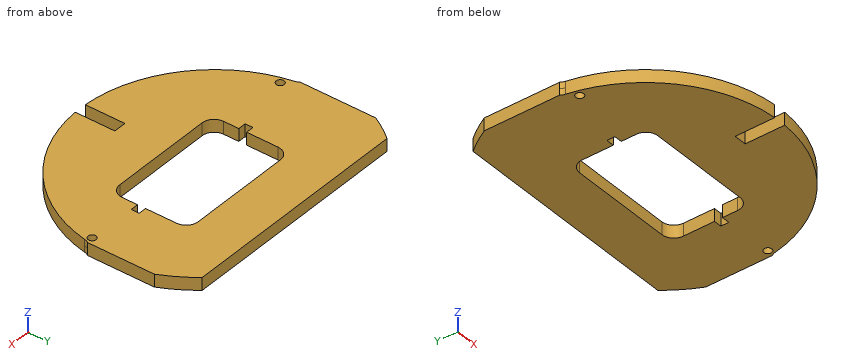
from build123d import *

# Parameters (mm, degrees)
BOSS_EXTRUDE1_DEPTH = 1.5875
SKETCH2_R           = 1
CUT_EXTRUDE1_DEPTH  = 3.175
SKETCH3_W           = 3.175
SKETCH3_H           = 10.970571453
CUT_EXTRUDE2_DEPTH  = 48.905462264
SKETCH4_W           = 2
SKETCH4_H           = 2
CUT_EXTRUDE3_DEPTH  = 48.879683973


with BuildPart() as part:
    # Sketch1 → Boss-Extrude1 (new, symmetric)
    with BuildSketch(Plane.XY):
        with BuildLine():
            Line((-29.861047016, 19.799597713), (28.798323584, 19.799597713))
            ThreePointArc((28.798323584, 19.799597713), (31.555543196, 15.909935232), (33.800017398, 11.703503281))
            Line((33.800017398, 11.703503281), (33.800017398, -5.129281896))
            add(Edge.make_bspline(
                [(33.333736062, -6.198908202), (33.370273649, -6.00495249), (33.420827163, -5.815771167), (33.570327065, -5.45389308), (33.6709127, -5.28028559), (33.800017398, -5.129281896)],
                knots=[0, 0, 0, 0, 0.5, 0.5, 1, 1, 1, 1], degree=3))
            ThreePointArc((33.333736062, -6.198908202), (-0.00068987, -33.79957838), (-33.333992426, -6.197552493))
            add(Edge.make_bspline(
                [(-33.800017403, -5.129281896), (-33.542046516, -5.431010319), (-33.407261527, -5.809359873), (-33.333992426, -6.197552493)],
                knots=[0, 0, 0, 0, 1, 1, 1, 1], degree=3))
            Line((-33.800017403, -5.129281896), (-33.800017403, 13.855371896))
            ThreePointArc((-33.800017403, 13.855371896), (-31.971328776, 16.92078434), (-29.861047016, 19.799597713))
        make_face()
    extrude(amount=BOSS_EXTRUDE1_DEPTH, both=True)

    # Sketch2 → Cut-Extrude1 (cut)
    with BuildSketch(Plane.XY.offset(1.5875)):
        with Locations((-31.216064399, -8.164436653)):
            Circle(SKETCH2_R)
        with Locations((32.009302375, -5.358989516)):
            Circle(SKETCH2_R)
    extrude(amount=-CUT_EXTRUDE1_DEPTH, mode=Mode.SUBTRACT)

    # Sketch3 → Cut-Extrude2 (cut, through all)
    with BuildSketch(Plane.XY.offset(1.5875)):
        with Locations((-0.013127042, -29.284890239)):
            Rectangle(SKETCH3_W, SKETCH3_H)
    extrude(amount=-CUT_EXTRUDE2_DEPTH, mode=Mode.SUBTRACT)

    # Sketch4 → Cut-Extrude3 (cut, through all)
    with BuildSketch(Plane.XY.offset(1.5875)):
        with BuildLine():
            Line((-14.257724699, 4.717183699), (-14.257724699, -8.984256283))
            ThreePointArc((-14.257724699, -8.984256283), (-13.379045042, -11.105576627), (-11.257724699, -11.984256283))
            Line((-11.257724699, -11.984256283), (14.878600613, -11.984256283))
            ThreePointArc((14.878600613, -11.984256283), (16.999920956, -11.105576627), (17.878600613, -8.984256283))
            Line((17.878600613, -8.984256283), (17.878600613, 4.717183699))
            ThreePointArc((17.878600613, 4.717183699), (16.999920956, 6.838504042), (14.878600613, 7.717183699))
            Line((14.878600613, 7.717183699), (-11.257724699, 7.717183699))
            ThreePointArc((-11.257724699, 7.717183699), (-13.379045042, 6.838504042), (-14.257724699, 4.717183699))
        make_face()
        with Locations((-15.257724699, -4.150157902)):
            Rectangle(SKETCH4_W, SKETCH4_H)
        with Locations((18.878600613, -4.150157902)):
            Rectangle(SKETCH4_W, SKETCH4_H)
    extrude(amount=-CUT_EXTRUDE3_DEPTH, mode=Mode.SUBTRACT)


solid = part.part
The model under review builds one solid part; all positions refer to its coordinate system, in mm. Give positions to 0.01 mm unless a question says otherwise; leave off trailing zeros. Order: outer loops, then holes, each group sorted by start corner. A loop starts at its lowest first (then second) coordinate and runs counter-clockwise, first axis right, second up. Notation, with made-up numbers: (73, -9.75) -> (83, -9.75) arc R16 cw to (83, -5.75) -> close; hole circle Ø9 at (77, -7). An arc over 180 degrees is marked (long way). Write item = value, one per line. Start each with the question number.
(1) For pin 1 Ø1.5 at (x, z) = (16, -0.5) entering from -Y; pin 2 Ø1 at (y, z) = (-27.5, 0.5) entering from -X; pin 3 Ø1 at (x, z) = (-15, 0) entering from -Y, all flat-tipped, find the tip position at first contact; note any pin that passes through.
(2) For L1, parallel to X at y = 4, z = -0.5; L2, parallel to Y at x = -4.5, z = -0.1; L3, parallel to Y at x = 2, z = 0.75, list the stretches that pass through material, from the lowest coordinate up. Write a range as from..to.
(3) Take a section at C-C (z = 0.5). State how many separate pieces and enclosed holes the cut face has, plus the area to 3 significant figures.
(4) Take a section at D-D (y = 16.5). Write out the cut boundary in (x, z), plus the area to 3 significant figures.
(5) Take a section at A-A (x = 16). Write out the cut boundary in (y, z), plus the area to 3 significant figures.
(6) Take a section at B-B (y = -25.5). Write out the cut boundary in (x, z).
Returned:
q1.pin_1 = -30.18
q1.pin_2 = -20.38
q1.pin_3 = -30.55
q2.L1 = -33.8..-14.26, 17.88..33.8
q2.L2 = -33.5..-11.98, 7.72..19.8
q2.L3 = -33.74..-11.98, 7.72..19.8
q3.separate_pieces = 1
q3.enclosed_holes = 3
q3.area = 2,440 mm²
q4.outline = (-32.25, -1.59) -> (31.18, -1.59) -> (31.18, 1.59) -> (-32.25, 1.59) -> close
q4.area = 201 mm²
q5.outline = (-29.79, -1.59) -> (-11.77, -1.59) -> (-11.77, 1.59) -> (-29.79, 1.59) -> close; (7.5, -1.59) -> (19.8, -1.59) -> (19.8, 1.59) -> (7.5, 1.59) -> close
q5.area = 96.3 mm²
q6.outline = (-22.23, -1.59) -> (-1.6, -1.59) -> (-1.6, 1.59) -> (-22.23, 1.59) -> close; (1.57, -1.59) -> (22.23, -1.59) -> (22.23, 1.59) -> (1.57, 1.59) -> close
